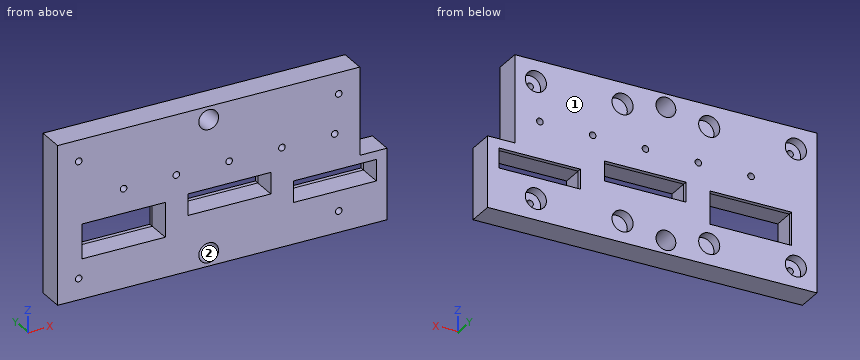
```python
from build123d import *

# Parameters (mm, degrees)
SKETCH1_W            = 229
SKETCH1_H            = 120
BOSS_EXTRUDE1_DEPTH  = 10
SKETCH4_W            = 20.632503002
SKETCH4_H            = 53.730004003
BOSS_EXTRUDE2_DEPTH  = 20
CUT_EXTRUDE1_REACH   = 239.573
SKETCH5_W            = 61.75
SKETCH5_H            = 15
SKETCH5_H_2          = 25
CUT_EXTRUDE2_REACH   = 239.573
SKETCH6_R            = 2.5
CUT_EXTRUDE3_REACH   = 239.573
SKETCH7_R            = 7.5
SKETCH8_R            = 8
CUT_EXTRUDE4_DEPTH   = 8
LPATTERN2_COUNT      = 4
LPATTERN2_PITCH      = 65.677
LPATTERN2_COUNT_DIR2 = 2
LPATTERN2_PITCH_DIR2 = 88
M6_TAPPED_HOLE2_D    = 5


with BuildPart() as part:
    # Sketch1 → Boss-Extrude1 (new, symmetric)
    with BuildSketch(Plane(origin=(0, 0, 0), x_dir=(1, 0, 0), z_dir=(0, 1, 0))):
        with Locations((-114.5, 0)):
            Rectangle(SKETCH1_W, SKETCH1_H)
    extrude(amount=BOSS_EXTRUDE1_DEPTH, both=True)

    # Sketch4 → Boss-Extrude2 (add)
    with BuildSketch(Plane(origin=(0, 10, 0), x_dir=(1, 0, 0), z_dir=(0, 1, 0))):
        with Locations((10.316251501, 33.134997999)):
            Rectangle(SKETCH4_W, SKETCH4_H)
    extrude(amount=-BOSS_EXTRUDE2_DEPTH)

    # Sketch5 → Cut-Extrude1 (cut, up to next)
    with BuildSketch(Plane(origin=(0, 10, 0), x_dir=(1, 0, 0), z_dir=(0, 1, 0)), mode=Mode.PRIVATE) as cut_extrude1_sk1:
        with Locations((-98.875, 9.852366083)):
            Rectangle(SKETCH5_W, SKETCH5_H)
    cut_extrude1_tool1 = extrude(cut_extrude1_sk1.sketch, amount=-CUT_EXTRUDE1_REACH, mode=Mode.PRIVATE) & part.part
    # Sketch5 → Cut-Extrude1 (cut, up to next)
    with BuildSketch(Plane(origin=(0, 10, 0), x_dir=(1, 0, 0), z_dir=(0, 1, 0)), mode=Mode.PRIVATE) as cut_extrude1_sk2:
        with Locations((-18.875, 20.69101)):
            Rectangle(SKETCH5_W, SKETCH5_H)
    cut_extrude1_tool2 = extrude(cut_extrude1_sk2.sketch, amount=-CUT_EXTRUDE1_REACH, mode=Mode.PRIVATE) & part.part
    # Sketch5 → Cut-Extrude1 (cut, up to next)
    with BuildSketch(Plane(origin=(0, 10, 0), x_dir=(1, 0, 0), z_dir=(0, 1, 0)), mode=Mode.PRIVATE) as cut_extrude1_sk3:
        with Locations((-178.875, 16.78)):
            Rectangle(SKETCH5_W, SKETCH5_H_2)
    cut_extrude1_tool3 = extrude(cut_extrude1_sk3.sketch, amount=-CUT_EXTRUDE1_REACH, mode=Mode.PRIVATE) & part.part
    add(cut_extrude1_tool1.solids().sort_by_distance((-98.875, 10, -9.852366))[0], mode=Mode.SUBTRACT)
    add(cut_extrude1_tool2.solids().sort_by_distance((-18.875, 10, -20.69101))[0], mode=Mode.SUBTRACT)
    add(cut_extrude1_tool3.solids().sort_by_distance((-178.875, 10, -16.78))[0], mode=Mode.SUBTRACT)

    # Sketch6 → Cut-Extrude2 (cut, up to next)
    with BuildSketch(Plane(origin=(0, 10, 0), x_dir=(1, 0, 0), z_dir=(0, 1, 0)), mode=Mode.PRIVATE) as cut_extrude2_sk1:
        with Locations(Location((-179, -14.72, 0), (0, 0, 270))):
            Circle(SKETCH6_R)
    cut_extrude2_tool1 = extrude(cut_extrude2_sk1.sketch, amount=-CUT_EXTRUDE2_REACH, mode=Mode.PRIVATE) & part.part
    # Sketch6 → Cut-Extrude2 (cut, up to next)
    with BuildSketch(Plane(origin=(0, 10, 0), x_dir=(1, 0, 0), z_dir=(0, 1, 0)), mode=Mode.PRIVATE) as cut_extrude2_sk2:
        with Locations(Location((-139, -14.72, 0), (0, 0, 270))):
            Circle(SKETCH6_R)
    cut_extrude2_tool2 = extrude(cut_extrude2_sk2.sketch, amount=-CUT_EXTRUDE2_REACH, mode=Mode.PRIVATE) & part.part
    # Sketch6 → Cut-Extrude2 (cut, up to next)
    with BuildSketch(Plane(origin=(0, 10, 0), x_dir=(1, 0, 0), z_dir=(0, 1, 0)), mode=Mode.PRIVATE) as cut_extrude2_sk3:
        with Locations(Location((-99, -14.72, 0), (0, 0, 270))):
            Circle(SKETCH6_R)
    cut_extrude2_tool3 = extrude(cut_extrude2_sk3.sketch, amount=-CUT_EXTRUDE2_REACH, mode=Mode.PRIVATE) & part.part
    # Sketch6 → Cut-Extrude2 (cut, up to next)
    with BuildSketch(Plane(origin=(0, 10, 0), x_dir=(1, 0, 0), z_dir=(0, 1, 0)), mode=Mode.PRIVATE) as cut_extrude2_sk4:
        with Locations(Location((-59, -14.72, 0), (0, 0, 270))):
            Circle(SKETCH6_R)
    cut_extrude2_tool4 = extrude(cut_extrude2_sk4.sketch, amount=-CUT_EXTRUDE2_REACH, mode=Mode.PRIVATE) & part.part
    # Sketch6 → Cut-Extrude2 (cut, up to next)
    with BuildSketch(Plane(origin=(0, 10, 0), x_dir=(1, 0, 0), z_dir=(0, 1, 0)), mode=Mode.PRIVATE) as cut_extrude2_sk5:
        with Locations(Location((-19, -14.72, 0), (0, 0, 270))):
            Circle(SKETCH6_R)
    cut_extrude2_tool5 = extrude(cut_extrude2_sk5.sketch, amount=-CUT_EXTRUDE2_REACH, mode=Mode.PRIVATE) & part.part
    add(cut_extrude2_tool1.solids().sort_by_distance((-179, 10, 14.72))[0], mode=Mode.SUBTRACT)
    add(cut_extrude2_tool2.solids().sort_by_distance((-139, 10, 14.72))[0], mode=Mode.SUBTRACT)
    add(cut_extrude2_tool3.solids().sort_by_distance((-99, 10, 14.72))[0], mode=Mode.SUBTRACT)
    add(cut_extrude2_tool4.solids().sort_by_distance((-59, 10, 14.72))[0], mode=Mode.SUBTRACT)
    add(cut_extrude2_tool5.solids().sort_by_distance((-19, 10, 14.72))[0], mode=Mode.SUBTRACT)

    # Sketch7 → Cut-Extrude3 (cut, up to next)
    with BuildSketch(Plane(origin=(0, 10, 0), x_dir=(1, 0, 0), z_dir=(0, 1, 0)), mode=Mode.PRIVATE) as cut_extrude3_sk1:
        with Locations(Location((-114.5, 50, 0), (0, 0, 270))):
            Circle(SKETCH7_R)
    cut_extrude3_tool1 = extrude(cut_extrude3_sk1.sketch, amount=-CUT_EXTRUDE3_REACH, mode=Mode.PRIVATE) & part.part
    # Sketch7 → Cut-Extrude3 (cut, up to next)
    with BuildSketch(Plane(origin=(0, 10, 0), x_dir=(1, 0, 0), z_dir=(0, 1, 0)), mode=Mode.PRIVATE) as cut_extrude3_sk2:
        with Locations(Location((-114.5, -50, 0), (0, 0, 270))):
            Circle(SKETCH7_R)
    cut_extrude3_tool2 = extrude(cut_extrude3_sk2.sketch, amount=-CUT_EXTRUDE3_REACH, mode=Mode.PRIVATE) & part.part
    add(cut_extrude3_tool1.solids().sort_by_distance((-114.5, 10, -50))[0], mode=Mode.SUBTRACT)
    add(cut_extrude3_tool2.solids().sort_by_distance((-114.5, 10, 50))[0], mode=Mode.SUBTRACT)

    # Draft1: read off the stored shape, not the designer's step
    # Draft1: loft between two sections, ruled curve by curve
    draft1_from = [
        Edge.make_line((-129.75, 6.8, -17.352366083), (-129.75, 6.8, -2.352366083)),
        Edge.make_line((-68, 6.8, -17.352366083), (-129.75, 6.8, -17.352366083)),
        Edge.make_line((-68, 6.8, -2.352366083), (-68, 6.8, -17.352366083)),
        Edge.make_line((-129.75, 6.8, -2.352366083), (-68, 6.8, -2.352366083)),
    ]
    draft1_to = [
        Edge.make_line((-130.336668927, -10, -17.93903501), (-130.336668927, -10, -1.765697156)),
        Edge.make_line((-67.413331073, -10, -17.93903501), (-130.336668927, -10, -17.93903501)),
        Edge.make_line((-67.413331073, -10, -1.765697156), (-67.413331073, -10, -17.93903501)),
        Edge.make_line((-130.336668927, -10, -1.765697156), (-67.413331073, -10, -1.765697156)),
    ]
    draft1 = Solid(Shell([*[Face.make_surface_from_curves(draft1_from[k], draft1_to[k]) for k in range(4)], Face(Wire(draft1_from)), Face(Wire(draft1_to))]))
    add(draft1, mode=Mode.SUBTRACT)

    # Draft1 2: loft between two sections, ruled curve by curve
    draft1_2_from = [
        Edge.make_line((-49.75, 6.8, -28.19101), (-49.75, 6.8, -13.19101)),
        Edge.make_line((12, 6.8, -28.19101), (-49.75, 6.8, -28.19101)),
        Edge.make_line((12, 6.8, -13.19101), (12, 6.8, -28.19101)),
        Edge.make_line((-49.75, 6.8, -13.19101), (12, 6.8, -13.19101)),
    ]
    draft1_2_to = [
        Edge.make_line((-50.336668927, -10, -28.777678927), (-50.336668927, -10, -12.604341073)),
        Edge.make_line((12.586668927, -10, -28.777678927), (-50.336668927, -10, -28.777678927)),
        Edge.make_line((12.586668927, -10, -12.604341073), (12.586668927, -10, -28.777678927)),
        Edge.make_line((-50.336668927, -10, -12.604341073), (12.586668927, -10, -12.604341073)),
    ]
    draft1_2 = Solid(Shell([*[Face.make_surface_from_curves(draft1_2_from[k], draft1_2_to[k]) for k in range(4)], Face(Wire(draft1_2_from)), Face(Wire(draft1_2_to))]))
    add(draft1_2, mode=Mode.SUBTRACT)

    # Draft1 3: loft between two sections, ruled curve by curve
    draft1_3_from = [
        Edge.make_line((-209.75, 6.8, -29.28), (-209.75, 6.8, -4.28)),
        Edge.make_line((-148, 6.8, -29.28), (-209.75, 6.8, -29.28)),
        Edge.make_line((-148, 6.8, -4.28), (-148, 6.8, -29.28)),
        Edge.make_line((-209.75, 6.8, -4.28), (-148, 6.8, -4.28)),
    ]
    draft1_3_to = [
        Edge.make_line((-210.336668927, -10, -29.866668927), (-210.336668927, -10, -3.693331073)),
        Edge.make_line((-147.413331073, -10, -29.866668927), (-210.336668927, -10, -29.866668927)),
        Edge.make_line((-147.413331073, -10, -3.693331073), (-147.413331073, -10, -29.866668927)),
        Edge.make_line((-210.336668927, -10, -3.693331073), (-147.413331073, -10, -3.693331073)),
    ]
    draft1_3 = Solid(Shell([*[Face.make_surface_from_curves(draft1_3_from[k], draft1_3_to[k]) for k in range(4)], Face(Wire(draft1_3_from)), Face(Wire(draft1_3_to))]))
    add(draft1_3, mode=Mode.SUBTRACT)

    # Sketch8 → Cut-Extrude4 (cut)
    with BuildSketch(Plane(origin=(0, 10, 0), x_dir=(1, 0, 0), z_dir=(0, 1, 0))):
        with Locations(Location((-213, 44, 0), (0, 0, 270))):
            Circle(SKETCH8_R)
    cut_extrude4 = extrude(amount=-CUT_EXTRUDE4_DEPTH, mode=Mode.SUBTRACT)

    # LPattern2: Cut-Extrude4 4 × 2
    with Locations(*[(i * LPATTERN2_PITCH, 0, j * LPATTERN2_PITCH_DIR2) for i in range(LPATTERN2_COUNT) for j in range(LPATTERN2_COUNT_DIR2) if (i, j) != (0, 0)]):
        add(cut_extrude4, mode=Mode.SUBTRACT)

    # M6 Tapped Hole2 (through all)
    with Locations(Plane(origin=(0, 2, 0), x_dir=(1, 0, 0), z_dir=(0, 1, 0))):
        with Locations((-213, 44), (-15.969, 44), (-15.969, -44), (-213, -44)):
            Hole(M6_TAPPED_HOLE2_D / 2)


solid = part.part
```
Geometry: final body of the model. Coordinates: model frame, mm. Face numbers are marked on the shaded views. Round coordinates to 2 decimals unless told otherwise and drop trailing zeros. Write each loop counter-clockwise with the first axis right and the second up, starting at its lowest first coordinate (ties: lowest second). Pieces come first, ordered by that corner, then holes. Notation, with made-up numbers: M 84,5 L 88,5 A13 cw 88,14 Z; hole C 23.25,25 d5. An arc over 180 degrees is marked long. Answer in a Markdown table with one row per item. Add a question column.
(1) Contact query for a flat-ended pin moving along its axis: pin 1 (8 mm diameter, centred on x = -145, z = 42.5, fed in from +Y). Output: stop coordinate, or through.
(2) Ray query, L1, parallel to X at y = 9, z = -8; L2, parallel to X at y = -0.5, z = 14.72; L3, parallel to Z at x = -213, y = -6.5. Return the intervals inside material, ascending.
(3) Cut plane C-C, the plane z = 14.72. Return the cut outline in (x, y).
(4) Cut plane D-D, the plane x = -114.5. Give the number of separate pieces and of enclosed holes in the cut face, then the cut area to 3 significant figures.
(5) Cut plane B-B, the plane x = -213. Return the cut outline in (y, z), then the cut area to 3 significant figures.
(6) Cut plane A-A, the plane x = -59. Return the cut outline in (y, z).
(7) Draft query along Z for the marked faces 1 and 2. Return one class per face: pulls with the +Z half, pulls with the -Z half, needs draft (parallel to the pull), parting line crosses it, or undercut.
Established:
| question | item | result |
|---|---|---|
| 1 | pin 1 | y = 2 |
| 2 | L1 | -229 to -209.75, -148 to -129.75, -68 to 20.63 |
| 2 | L2 | -229 to -181.5, -176.5 to -141.5, -136.5 to -101.5, -96.5 to -61.5, -56.5 to -21.5, -16.5 to 0 |
| 2 | L3 | -60 to -46.5, -41.5 to 41.5, 46.5 to 60 |
| 3 | outline | M -229,-10 L -181.5,-10 L -181.5,10 L -229,10 Z; M -176.5,-10 L -141.5,-10 L -141.5,10 L -176.5,10 Z; M -136.5,-10 L -101.5,-10 L -101.5,10 L -136.5,10 Z; M -96.5,-10 L -61.5,-10 L -61.5,10 L -96.5,10 Z; M -56.5,-10 L -21.5,-10 L -21.5,10 L -56.5,10 Z; M -16.5,-10 L 0,-10 L 0,10 L -16.5,10 Z |
| 4 | separate pieces | 4 |
| 4 | enclosed holes | 0 |
| 4 | area | 1,490 mm² |
| 5 | outline | M -10,-60 L 10,-60 L 10,-52 L 2,-52 L 2,-46.5 L -10,-46.5 Z; M -10,-41.5 L 2,-41.5 L 2,-36 L 10,-36 L 10,36 L 2,36 L 2,41.5 L -10,41.5 Z; M -10,46.5 L 2,46.5 L 2,52 L 10,52 L 10,60 L -10,60 Z |
| 5 | area | 2,020 mm² |
| 6 | outline | M -10,-60 L 10,-60 L 10,12.22 L -10,12.22 Z; M -10,17.22 L 10,17.22 L 10,60 L -10,60 Z |
| 7 | face 1 | needs draft |
| 7 | face 2 | undercut |
